Verification items for this drawing (mm, ordinates from the low corner). A direction names the side the tool comes from. Give positions to 0.01 mm unless a question says otherwise; leave off trailing zeros. Loops run counter-clockwise (first coordinate to the right, second up) from the corner with the lowest first, then second, coordinate; pieces in that order, holes last. Notation, with made-up numbers: M 16.25,-11 L 33.25,-11 A36 cw 33.25,23 Z; hole C -35,19 d6. An arc over 180 degrees is marked long. Use one line per item in the form item = value.
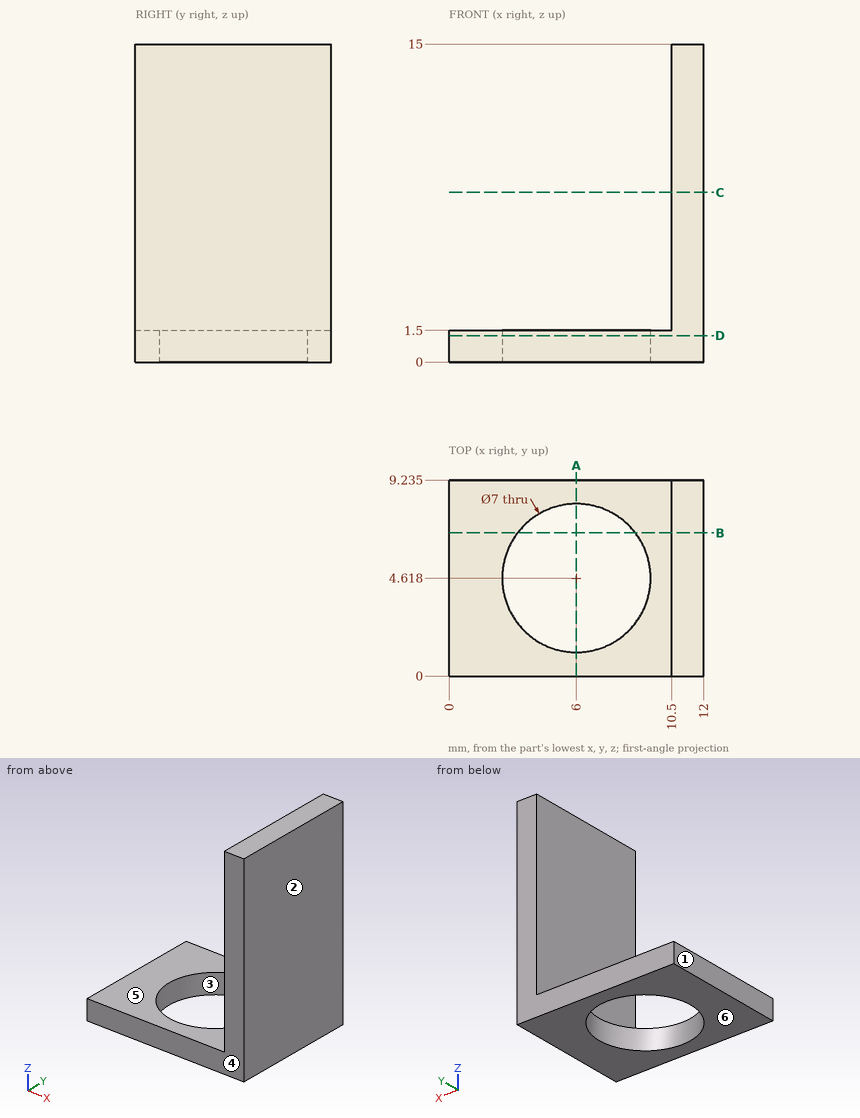
1) Section check D-D (z = 1.25). Record the cut outline in (x, y) (1 decimal).
Evaluation:
outline = M 0,0 L 12,0 L 12,9.2 L 0,9.2 Z; hole C 6,4.6 d7
2) Set-up check for the marked faces 5 and 6: record each of +Z, -Z, +X, -X, +Y, -Y from which the full face is reachable in a straight line by a thin tool's end or side.
Evaluation:
face_5 = +Z, -X, +Y, -Y
face_6 = -Z, +X, -X, +Y, -Y
3) Section check A-A (x = 6). Record the cut outline in (y, z) (1 decimal).
Evaluation:
outline = M 0,0 L 1.1,0 L 1.1,1.5 L 0,1.5 Z; M 8.1,0 L 9.2,0 L 9.2,1.5 L 8.1,1.5 Z
4) Section check B-B (y = 6.75). Record the cut outline in (x, z) (1 decimal).
Evaluation:
outline = M 0,0 L 3.2,0 L 3.2,1.5 L 0,1.5 Z; M 8.8,0 L 12,0 L 12,15 L 10.5,15 L 10.5,1.5 L 8.8,1.5 Z
5) Scan lines: line 1 (Y direction, x = 6, z = 0.8) (1 decimal); line 2 (Z direction, x = 10.25, y = 0.75); line 3 (X direction, y = 3.5, z = 7.25). Record each from-to range of solid material in increasing order.
Evaluation:
line_1 = 0 to 1.1, 8.1 to 9.2
line_2 = 0 to 1.5
line_3 = 10.5 to 12
6) Release check for a two-part mould opening along X. For the marked faces 1, 2, 3 and 4 record: pulls with the +X half, pulls with the -X half, needs draft (parallel to the pull), parting line crosses it, or undercut.
Evaluation:
face_1 = pulls with the -X half
face_2 = pulls with the +X half
face_3 = undercut
face_4 = needs draft
7) Section check C-C (z = 8). Record the cut outline in (x, y) (1 decimal).
Evaluation:
outline = M 10.5,0 L 12,0 L 12,9.2 L 10.5,9.2 Z
8) Depth check by flat-ended pin: pin 1 Ø5 at (x, z) = (5, 5.5) entering from +Y; pin 2 Ø5 at (x, y) = (8.5, 8) entering from +Z. Enter the tip coordinate at first touch or a pass-through.
Evaluation:
pin_1 = through
pin_2 = 15
